The model under review builds one solid part; all positions refer to its coordinate system, in mm. A direction names the side the tool comes from. Coordinates: 2 decimals unless noted, no trailing zeros. Write each loop counter-clockwise with the first axis right and the second up, starting at its lowest first coordinate (ties: lowest second). Pieces come first, ordered by that corner, then holes. Notation, with made-up numbers: (51, 21.5) -> (89, 21.5) arc R21 ccw to (89, 57.5) -> close; hole circle Ø2 at (-10.75, 81.5). An arc over 180 degrees is marked (long way). Put each result on its own line as item: value. Start each with the question number.
from build123d import *

# Parameters (mm, degrees)
BOSS_EXTRUDE1_DEPTH = 75
SKETCH2_R           = 1.75
CUT_EXTRUDE1_DEPTH  = 25
SKETCH4_R           = 1.75
CUT_EXTRUDE3_DEPTH  = 25
SKETCH5_R           = 2.1
CUT_EXTRUDE4_DEPTH  = 10


with BuildPart() as part:
    # Sketch1 → Boss-Extrude1 (new body)
    with BuildSketch(Plane.XY):
        Polygon((-20, 159.45), (-20, 13), (0, 13), (1, 13), (1, 94.5), (-1.5, 94.5), (-1.5, 159.45), align=None)
    extrude(amount=BOSS_EXTRUDE1_DEPTH)

    # Sketch2 → Cut-Extrude1 (cut)
    with BuildSketch(Plane(origin=(1, 0, 0), x_dir=(0, 0, -1), z_dir=(1, 0, 0))):
        with Locations((-37.5, 18.5)):
            Circle(SKETCH2_R)
    extrude(amount=-CUT_EXTRUDE1_DEPTH, mode=Mode.SUBTRACT)

    # Sketch4 → Cut-Extrude3 (cut)
    with BuildSketch(Plane(origin=(-1.5, 0, 0), x_dir=(0, 0, -1), z_dir=(1, 0, 0))):
        with Locations((-37.5, 107.5)):
            Circle(SKETCH4_R)
    extrude(amount=-CUT_EXTRUDE3_DEPTH, mode=Mode.SUBTRACT)

    # Sketch5 → Cut-Extrude4 (cut)
    with BuildSketch(Plane.XZ.offset(-13)):
        with Locations(Location((-9.5, 50, 0), (0, 0, 270))):
            Circle(SKETCH5_R)
        with Locations(Location((-9.5, 25, 0), (0, 0, 270))):
            Circle(SKETCH5_R)
    extrude(amount=-CUT_EXTRUDE4_DEPTH, mode=Mode.SUBTRACT)


solid = part.part
1. Insertion check: P1, Ø19.5, axis at y = 126.5, z = 26, coming from the +X side; P2, Ø4, axis at x = -9.5, z = 50, coming from the -Y side; P3, Ø6.5, axis at x = -9.5, z = 25, coming from the -Y side. Each pin has a flat end and moves straight along its axis. Give the tip position at first contact, or say it passes through.
2. Tool access review of faces 1 (the flat face through (0, 94.5, 37)), 2 (the flat face through (-9, 23, 50)), 3 (the flat face through (-10, 13, 37)): name each direction out of +Z, -Z, +X, -X, +Y, -Y from which nothing blocks a thin tool from reaching the whole face with its end or side.
3. The part is to be moulded in two halves that separate along Z. For faces 4 (the cylindrical face through (-7.418, 17.93, 25.273)), 5 (the flat face through (1, 53, 37)), 6 (the cylindrical face through (-8.869, 17.93, 47.997)), 7 (the flat face through (-10, 87, 0)), say which applies: released by +Z, released by -Z, zero draft, split by the parting line, or undercut.
4. Consider section A-A on y = 18.5. State the section outline as (x, z) points, then the cut area to 3 significant figures.
5. Consider section B-B on z = 37.5. State the section outline as (x, y) points.
6. Consider section D-D on z = 25. State the section outline as (x, y) points, then the cut area to 3 significant figures.
7. Consider section C-C on y = 107.5. State the section outline as (x, z) points.
8. Wall thickness on line 1 (Y direction, x = -10.75, z = 37.5); line 2 (X direction, y = 17.25, z = 25); line 3 (Z direction, x = -16, y = 107.5): over which ranges is each line inside the solid? List them lowest first. Write a range as from..to.
Output values:
1. P1: stops at x = -1.5
1. P2: stops at y = 23
1. P3: stops at y = 13
2. face 1: +Z, -Z, +X, +Y
2. face 2: -Y
2. face 3: +Z, -Z, +X, -X, -Y
3. face 4: undercut
3. face 5: zero draft
3. face 6: undercut
3. face 7: released by -Z
4. outline: (-20, 0) -> (1, 0) -> (1, 35.75) -> (-20, 35.75) -> close; (-20, 39.25) -> (1, 39.25) -> (1, 75) -> (-20, 75) -> close; hole circle Ø4.2 at (-9.5, 25); hole circle Ø4.2 at (-9.5, 50)
4. area: 1,470 mm^2
5. outline: (-20, 13) -> (1, 13) -> (1, 16.75) -> (-20, 16.75) -> close; (-20, 20.25) -> (1, 20.25) -> (1, 94.5) -> (-1.5, 94.5) -> (-1.5, 105.75) -> (-20, 105.75) -> close; (-20, 109.25) -> (-1.5, 109.25) -> (-1.5, 159.45) -> (-20, 159.45) -> close
6. outline: (-20, 13) -> (-11.6, 13) -> (-11.6, 23) -> (-7.4, 23) -> (-7.4, 13) -> (1, 13) -> (1, 94.5) -> (-1.5, 94.5) -> (-1.5, 159.45) -> (-20, 159.45) -> close
6. area: 2,870 mm^2
7. outline: (-20, 0) -> (-1.5, 0) -> (-1.5, 35.75) -> (-20, 35.75) -> close; (-20, 39.25) -> (-1.5, 39.25) -> (-1.5, 75) -> (-20, 75) -> close
8. line 1: y = 13..16.75, 20.25..105.75, 109.25..159.45
8. line 2: x = -20..-11.6, -7.4..1
8. line 3: z = 0..35.75, 39.25..75
